Work out the finished part from the listing and answer in its coordinate system (mm). A direction names the side the tool comes from. Round coordinates to 2 decimals unless told otherwise and drop trailing zeros. Write each loop counter-clockwise with the first axis right and the second up, starting at its lowest first coordinate (ties: lowest second). Pieces come first, ordered by that corner, then holes.
from build123d import *

# Parameters (mm, degrees)
SKETCH1_R           = 14.2875
SKETCH1_R_2         = 6.35
BOSS_EXTRUDE1_DEPTH = 10.31875
CUT_EXTRUDE1_DEPTH  = 10.31875
CUT_EXTRUDE2_DEPTH  = 10.31875


with BuildPart() as part:
    # Sketch1 → Boss-Extrude1 (new body)
    with BuildSketch(Plane(origin=(0, 0, 0), x_dir=(1, 0, 0), z_dir=(0, 1, 0))):
        Circle(SKETCH1_R)
        Circle(SKETCH1_R_2, mode=Mode.SUBTRACT)
    extrude(amount=BOSS_EXTRUDE1_DEPTH)

    # Sketch2 → Cut-Extrude1 (cut)
    with BuildSketch(Plane(origin=(0, 0, 0), x_dir=(0, 0, -1), z_dir=(1, 0, 0))):
        with BuildLine():
            Line((-14.2875, 7.944437688), (-16.071181414, 7.944437688))
            Line((-16.071181414, 7.944437688), (-16.071181414, 2.435187999))
            Line((-16.071181414, 2.435187999), (-14.2875, 2.435187999))
            ThreePointArc((-14.2875, 2.435187999), (-11.532875155, 5.189812844), (-14.2875, 7.944437688))
        make_face()
    extrude(amount=-CUT_EXTRUDE1_DEPTH, mode=Mode.SUBTRACT)

    # Sketch3 → Cut-Extrude2 (cut)
    with BuildSketch(Plane(origin=(0, 10.31875, 0), x_dir=(1, 0, 0), z_dir=(0, 1, 0))):
        with BuildLine():
            Line((0, -6.35), (0, -14.2875))
            ThreePointArc((0, -14.2875), (-0.747749975, -14.267919478), (-1.493450419, -14.20923158))
            Line((-1.493450419, -14.20923158), (-0.663755742, -6.315214036))
            ThreePointArc((-0.663755742, -6.315214036), (-0.332333322, -6.341297546), (0, -6.35))
        make_face()
    extrude(amount=-CUT_EXTRUDE2_DEPTH, mode=Mode.SUBTRACT)


solid = part.part
Q1. The mould has two halves that part along X. Classify faces 1 (the face through (0, 10.319, -7)), 2 (the face through (-0.992, 5.232, 9.44)), 3 (the face through (0, 5, 10)): +X half, -X half, draft (parallel to the pull), parting line (faces both ways), or undercut.
Q2. A tool of negligible diameter and unlimited length cuts with its end or side. For faces 4 (the face through (0, 0, -7)), 5 (the face through (-3.935, 5.13, 11.534)), from which of +Z, -Z, +X, -X, +Y, -Y can it reach the whole face along a straight path? Write none if from no direction.
Q3. Find the intervals of material crossed by L1, parallel to X at y = 4.25, z = 0; L2, parallel to X at y = 7.25, z = 9.75; L3, parallel to Z at x = 2.5, y = 4.5, in increasing order.
Q4. Given pin 1 (11.5 mm diameter, centred on x = 0, z = 0, fed in from +Y); pin 2 (2 mm diameter, centred on x = 11, y = 1.5, fed in from -Z); pin 3 (3 mm diameter, centred on y = 6.5, z = 8.5, fed in from -X); pin 4 (1.5 mm diameter, centred on y = 3, z = 1.5, fed in from +X), each flat-ended and moving along its own axis, determine where each tip first touches the part or whether it passes through.
Q5. Find section A-A (z = 4.5). Determine the outline of the cut face in (x, y).
Q6. Find section B-B (x = 2). Determine the outline of the cut face in (y, z), plus the area to 3 significant figures.
Report:
1. face 1: draft
1. face 2: undercut
1. face 3: undercut
2. face 4: +Z, -Z, +X, -X, -Y
2. face 5: +Z, -X
3. L1: x = -14.29 to -6.35, 6.35 to 14.29
3. L2: x = -10.44 to -1.02, 0 to 10.44
3. L3: z = -14.07 to -5.84, 5.84 to 14.07
4. pin 1: passes through
4. pin 2: stops at z = -10.2
4. pin 3: stops at x = -12.46
4. pin 4: stops at x = 14.27
5. outline: (-13.56, 0) - (-4.48, 0) - (-4.48, 10.32) - (-13.56, 10.32) - close; (4.48, 0) - (13.56, 0) - (13.56, 10.32) - (4.48, 10.32) - close
6. outline: (0, -14.15) - (10.32, -14.15) - (10.32, -6.03) - (0, -6.03) - close; (0, 6.03) - (10.32, 6.03) - (10.32, 14.15) - (0, 14.15) - close
6. area: 168 mm2
